from build123d import *

# Parameters (mm, degrees)
SKETCH_1_R      = 1.55
EXTRUDE_1_DEPTH = 4


with BuildPart() as part:
    # 草圖1 → 填料-伸長1 (new body)
    with BuildSketch(Plane(origin=(0, 4, 0), x_dir=(1, 0, 0), z_dir=(0, 1, 0))):
        Polygon((-4, 7), (-4, 15), (-12, 15), (-12, -7), (-4, -7), (-4, -15), (4, -15), (4, -7), (12, -7), (12, 15), (4, 15), (4, 7), align=None)
        Circle(SKETCH_1_R, mode=Mode.SUBTRACT)
    extrude(amount=-EXTRUDE_1_DEPTH)


solid = part.part
Work out the finished part from the listing and answer in its coordinate system (mm). A direction names the side the tool comes from. Give positions to 0.01 mm unless a question says otherwise; leave off trailing zeros. Loops run counter-clockwise (first coordinate to the right, second up) from the corner with the lowest first, then second, coordinate; pieces in that order, holes last. Notation, with made-up numbers: (65.25, 5) -> (105.25, 5) arc R17 ccw to (105.25, 15) -> close; hole circle Ø3 at (76, -29). An arc over 180 degrees is marked (long way). Use a Markdown table: item, result. Add a question column.
1. Flat-ended cylindrical pins translate along their axes: pin 1 Ø1.2 at (x, y) = (-9.5, 2) entering from +Z; pin 2 Ø2 at (y, z) = (2, 9.5) entering from +X. Find the tip coordinate at first contact, or state that the pin passes through.
2. Section C-C on x = 0 is taken. Determine the outline of the cut face in (y, z), and give its area (3 significant figures).
3. For faces 5 (the flat face through (12, 2, -4)), 6 (the flat face through (-8, 2, -15)), 7 (the flat face through (-8, 2, 7)), 8 (the flat face through (0, 2, -7)), 9 (the flat face through (8, 2, 7)), determine the directions among +Z, -Z, +X, -X, +Y, -Y from which every point of the face is accessible in a straight line to the end or side of a thin tool.
4. Find the intervals of material crossed by probe 1 along X at (y, z) = (1.6, 0); probe 2 along X at (y, z) = (2.9, -10); probe 3 along Z at (x, y) = (0, 2.7), in increasing order.
5. Determine the mould class of faces 1 (the flat face through (-4, 2, -11)), 2 (the flat face through (4, 2, 11)), 3 (the flat face through (4, 2, -11)), 4 (the flat face through (0, 0, -4)) for opening direction X: released by +X, released by -X, zero draft, split by the parting line, or undercut.
6. Section A-A on y = 2.55 is taken. Determine the outline of the cut face in (x, z).
7. Section B-B on z = 0 is taken. Determine the outline of the cut face in (x, y).
Results below:
| question | item | result |
|---|---|---|
| 1 | pin 1 | stops at z = 7 |
| 1 | pin 2 | stops at x = 4 |
| 2 | outline | (0, -7) -> (4, -7) -> (4, -1.55) -> (0, -1.55) -> close; (0, 1.55) -> (4, 1.55) -> (4, 15) -> (0, 15) -> close |
| 2 | area | 75.6 mm^2 |
| 3 | face 5 | +Z, -Z, +X, +Y, -Y |
| 3 | face 6 | -Z, +X, -X, +Y, -Y |
| 3 | face 7 | +Z, -X, +Y, -Y |
| 3 | face 8 | -Z, +Y, -Y |
| 3 | face 9 | +Z, +X, +Y, -Y |
| 4 | probe 1 | x = -12 to -1.55, 1.55 to 12 |
| 4 | probe 2 | x = -12 to -4, 4 to 12 |
| 4 | probe 3 | z = -7 to -1.55, 1.55 to 15 |
| 5 | face 1 | undercut |
| 5 | face 2 | released by +X |
| 5 | face 3 | undercut |
| 5 | face 4 | zero draft |
| 6 | outline | (-12, -15) -> (-4, -15) -> (-4, -7) -> (4, -7) -> (4, -15) -> (12, -15) -> (12, 7) -> (4, 7) -> (4, 15) -> (-4, 15) -> (-4, 7) -> (-12, 7) -> close; hole circle Ø3.1 at (0, 0) |
| 7 | outline | (-12, 0) -> (-1.55, 0) -> (-1.55, 4) -> (-12, 4) -> close; (1.55, 0) -> (12, 0) -> (12, 4) -> (1.55, 4) -> close |
